Verification items for the finished model (mm, model axes). A direction names the side the tool comes from. Give positions to 0.01 mm unless a question says otherwise; leave off trailing zeros. Loops run counter-clockwise (first coordinate to the right, second up) from the corner with the lowest first, then second, coordinate; pieces in that order, holes last. Notation, with made-up numbers: M -1.5,10.5 L 24.5,10.5 A24 cw 24.5,33.5 Z; hole C 45.5,17.25 d8. An arc over 180 degrees is marked long. Put each result on its own line as item: value. Start each with the question number.
Autodesk Inventor part; units mm, degrees
ref_plane "YZ Plane" through (0, 0, 0) normal (1, 0, 0) x (0, 1, 0)
ref_plane "XZ Plane" through (0, 0, 0) normal (0, 1, 0) x (-1, 0, 0)
ref_plane "XY Plane" through (0, 0, 0) normal (0, 0, 1) x (1, 0, 0)
sketch "Sketch1" plane through (0, 0, 0) normal (0, 0, 1) x (1, 0, 0)
  line L0 (0, 35) -> (0, 0)
  line L1 (0, 0) -> (35, 0)
  line L2 (35, 0) -> (35, 6)
  line L3 (35, 6) -> (6, 6)
  line L4 (6, 6) -> (6, 35)
  line L5 (6, 35) -> (0, 35)
  line L6 (6, 25) -> (25, 6)
  line L7 (6, 16.5147) -> (16.5147, 6)
  dimension "d0" = 6
  dimension "d1" = 35
  dimension "d5" = 45
  dimension "d6" = 10
  dimension "d24" = 6
extrude "Extrusion1" add sketch "Sketch1" along normal blind 10 contours L5 L4 L3 L2 L1 L0 | L6 L3 L7 L4
sketch "Sketch2" plane through (0, 0, 0) normal (0, -1, 0) x (1, 0, 0)
  line L0 (35, 0) -> (35, 10)
  point P0 (0, 0)
  point P1 (30, 5)
  point P2 (10, 5)
  point P3 (35, 5)
  dimension "d7" = 5
  dimension "d8" = 20
hole "Hole1" at (30, 0, 5) at (10, 0, 5) direction (0, 1, 0) diameter 4 depth 8
sketch "Sketch3" plane through (0, 0, 0) normal (-1, 0, 0) x (0, 0, 1)
  line L0 (0, 35) -> (10, 35)
  line L1 (0, 0) -> (10, 0)
  point P0 (5, 31.5)
  point P1 (5, 35)
  dimension "d16" = 31.5
hole "Hole2" at (0, 31.5, 5) direction (1, 0, 0) diameter 4 depth 8
fillet "Fillet1" radius 1 10 edges at (0, 35, 5) (6, 35, 5) (0, 0, 5) (35, 0, 5) (35, 6, 5) (25, 6, 5) (6, 25, 5) (6, 6, 5) (6, 16.5147, 5) (16.5147, 6, 5)
chamfer "Chamfer1" distance 1 angle 45 36 edges at (0, 17.5, 10) (0.2929, 0.2929, 10) (17.5, 0, 10) (34.7071, 0.2929, 10) (35, 3, 10) (34.7071, 5.7071, 10) (29.7071, 6, 10) (25.0315, 6.0761, 10) (15.5, 15.5, 10) (6.0761, 25.0315, 10) (6, 29.7071, 10) (5.7071, 34.7071, 10) (3, 35, 10) (0.2929, 34.7071, 10) (11.2574, 11.2574, 10) (10.5503, 6, 10) (6.2929, 6.2929, 10) (6, 10.5503, 10) (6, 10.5503, 0) (11.2574, 11.2574, 0) (10.5503, 6, 0) (6.2929, 6.2929, 0) (0, 17.5, 0) (0.2929, 0.2929, 0) (17.5, 0, 0) (34.7071, 0.2929, 0) (35, 3, 0) (34.7071, 5.7071, 0) (29.7071, 6, 0) (25.0315, 6.0761, 0) (15.5, 15.5, 0) (6.0761, 25.0315, 0) (6, 29.7071, 0) (5.7071, 34.7071, 0) (3, 35, 0) (0.2929, 34.7071, 0)
properties part number "Control Board Bracket"
Q1. Go/stop test with flat-tipped pins: pin 1 (3 mm diameter, centred on y = 23.5, z = 7, fed in from +X); pin 2 (3.5 mm diameter, centred on y = 9.5, z = 5, fed in from +X); pin 3 (3.5 mm diameter, centred on x = 9, z = 6, fed in from +Y). Record where each tip stops, or that it passes through.
Q2. Release check for a two-part mould opening along Y. For faces 1 (the face through (11.556, 11.655, 9.493)), 2 (the face through (0.285, 0.301, 5.056)), 3 (the face through (5.355, 34.363, 9.493)) record: pulls with the +Y half, pulls with the -Y half, needs draft (parallel to the pull), parting line crosses it, or undercut.
Q3. Cross-section at A-A, the plane x = 30. Record the boundary of the cut face in (y, z).
Q4. Cross-section at D-D, the plane z = 6.5. State how many separate pieces and enclosed holes the cut face has, then the cut area to 3 significant figures.
Q5. Set-up check for faces 4 (the face through (6, 29, 5)), 5 (the face through (8, 3, 5)), 6 (the face through (15.399, 6.487, 0.604)): record each of +Z, -Z, +X, -X, +Y, -Y from which the full face is reachable in a straight line by a thin tool's end or side.
Q6. Scan lines: L1, parallel to X at y = 4.05, z = 5; L2, parallel to Z at x = 1.6, y = 31.5; L3, parallel to Y at x = 2.2, z = 5. Record each from-to range of solid material in increasing order.
Q7. Cross-section at B-B, the plane z = 1.75. Record the boundary of the cut face in (x, y), then the cut area to 3 significant figures.
Ans:
1. pin 1: stops at x = 9
1. pin 2: stops at x = 23.25
1. pin 3: stops at y = 23.75
2. face 1: undercut
2. face 2: pulls with the -Y half
2. face 3: pulls with the +Y half
3. outline: M 0,1 L 1,0 L 5,0 L 6,1 L 6,3 L 0,3 Z; M 0,7 L 6,7 L 6,9 L 5,10 L 1,10 L 0,9 Z
4. separate pieces: 3
4. enclosed holes: 0
4. area: 463 mm^2
5. face 4: +Z, -Z, +X, +Y
5. face 5: -Y
5. face 6: -Z
6. L1: x = 0 to 8, 12 to 28, 32 to 35
6. L2: z = 0 to 3, 7 to 10
6. L3: y = 0 to 29.5, 33.5 to 35
7. outline: M 0,1 A1 ccw 1,0 L 34,0 A1 ccw 35,1 L 35,5 A1 ccw 34,6 L 25.41,6 A1 cw 24.71,6.29 L 6.29,24.71 A1 cw 6,25.41 L 6,34 A1 ccw 5,35 L 1,35 A1 ccw 0,34 Z; hole M 6,7 A1 ccw 7,6 L 14.1,6 A1 ccw 14.81,7.71 L 7.71,14.81 A1 ccw 6,14.1 Z
7. area: 511 mm^2
